Autodesk Inventor part; units mm, degrees
ref_plane "Work Plane1" through (1.525, 0, 0) normal (0, 0, 1) x (1, 0, 0)
ref_plane "YZ Plane" through (0, 0, 0) normal (1, 0, 0) x (0, 1, 0)
ref_plane "XZ Plane" through (0, 0, 0) normal (0, 1, 0) x (-1, 0, 0)
sketch "Sketch1" plane through (0, 0, 0) normal (0, 0, 1) x (1, 0, 0)
  line L0 (0, 10) -> (80, 10)
  line L1 (80, 10) -> (80, 0)
  line L2 (80, 0) -> (0, 0)
  line L3 (-16, 0) -> (96, 0)
  line L4 (0, -2) -> (0, 12)
  line L5 (0, 10) -> (0, 0)
  dimension "d2" = 20
  dimension "d59" = 80
revolve "Body" add sketch "Sketch1" angle 360 about axis through (80, 0, 0) along (-1, 0, 0)
sketch "Sketch2" plane through (0, 0, 0) normal (-1, 0, 0) x (0, 0, 1)
  line L0 (0, 17.3205) -> (15, 8.6603)
  line L1 (15, 8.6603) -> (15, -8.6603)
  line L2 (15, -8.6603) -> (0, -17.3205)
  line L3 (0, -17.3205) -> (-15, -8.6603)
  line L4 (-15, -8.6603) -> (-15, 8.6603)
  line L5 (-15, 8.6603) -> (0, 17.3205)
  line L6 (-21, 0) -> (21, 0)
  line L7 (0, 24.2487) -> (0, -24.2487)
  point P0 (0, 0)
  point P1 (0, 0)
  dimension "d11" = 30
extrude "Head" add sketch "Sketch2" along normal blind 13.4
sketch "Sketch4" plane through (0, 0, 0) normal (0, 0, 1) x (1, 0, 0)
  line L0 (-11.6679, 18) -> (-13.4, 15)
  line L1 (-1.1, 0) -> (-0.234, 0)
  line L2 (-16.0332, 0) -> (2.3992, 0)
  line L3 (-13.4, 18) -> (-11.6679, 18)
  line L4 (-13.4, 15) -> (-13.4, 18)
  line L5 (0, 21.6) -> (0, -3.6)
  dimension "d65" = 30
  dimension "d67" = 30
  dimension "d68" = 36
  dimension "d69" = 13.4
revolve "Chamfer1" cut sketch "Sketch4" angle 360 about axis through (-1.1, 0, 0) along (1, 0, 0)
thread "Thread"
chamfer "Chamfer2" distance 1.5336 distance2 1.5337 1 edges at (80, -10, 0) measured on face at (80, -2.8768, 3.7595)
fillet "Fillet" radius 0.8 1 edges at (0, -10, 0)
ref_plane "Work Plane1" through (1.525, 0, 0) normal (0, 0, 1) x (1, 0, 0)
equation "\"d2\" = GD"
equation "\"d59\" = NLG"
equation "\"d11\" = SW"
equation "\"d3\" = KOH"
equation "\"d15\" = GEL"
equation "\"d6\" = -0.5 * SPD + 0.5 * GD"
equation "\"d71\" = RR1"
equation "\"d65\" = SW"
equation "\"d67\" = ANG1"
equation "\"d68\" = 1.2 * SW"
equation "\"d69\" = KOH"
equation "\"NLG\" = 80"
equation "\"GD\" = NND"
equation "\"KOH\" = 13.4"
equation "\"GEL\" = 46"
equation "\"SW\" = 30"
equation "\"SPD\" = NND - 1.2269 * PTC"
equation "\"SD\" = 0"
equation "\"ANG1\" = 30deg"
equation "\"GAL\" = 0.61345 * PTC"
equation "\"GUL\" = 0.61345 * PTC"
equation "\"RR\" = 0.1"
equation "\"RR1\" = 0.8"
equation "\"GD1\" = THREADDIA - 1.2269 * PTC"
equation "\"TOA\" = 30deg"
equation "\"PTC\" = 2.5"
equation "\"KOH1\" = 8.8"
equation "\"E0\" = 1.155 * SW"
properties part number "ANSI B18.2.3.5M - M20 x 2,5 x 80" material "Steel, Mild"
For this review, take the finished solid that the model builds, in its own axes (mm). A direction names the side the tool comes from. Round coordinates to 2 decimals unless told otherwise and drop trailing zeros. Loops run counter-clockwise (first coordinate to the right, second up) from the corner with the lowest first, then second, coordinate; pieces in that order, holes last. Notation, with made-up numbers: (49.5, -23.5) - (95.5, -23.5) arc R32 cw to (95.5, 6.5) - close; hole circle Ø6 at (46, 21). An arc over 180 degrees is marked (long way). One line per question, with ' | ' between items.
Q1. Tool access review of faces 1 (the flat face through (-6.606, -13.051, -7.395)), 2 (the cylindrical face through (40.18, -2.17, -9.76)): name each direction out of +Z, -Z, +X, -X, +Y, -Y from which nothing blocks a thin tool from reaching the whole face with its end or side.
Taken from the geometry:
face 1: -Z, +X, -X, -Y | face 2: +X
Q2. For pin 1 (4 mm diameter, centred on x = 15.5, z = 2, fed in from +Y); pin 2 (4 mm diameter, centred on x = 47, z = 10, fed in from +Y); pin 3 (1.5 mm diameter, centred on x = 57, z = 4.5, fed in from -Y), all flat-tipped, find the tip position at first contact; note any pin that passes through.
Taken from the geometry:
pin 1: stops at y = 10 | pin 2: stops at y = 6 | pin 3: stops at y = -9.27
Q3. Take a section at A-A (x = 47). Give the boundary of the cut face in (y, z), and give its area (3 significant figures).
Taken from the geometry:
outline: circle Ø20 at (0, 0) | area: 314 mm²
Q4. For line 1 along Y through (x, z) = (63, -0.5); line 2 along X through (y, z) = (-9.5, 6.5); line 3 along Z through (x, y) = (69.5, -5), list the stretches that pass through material, from the lowest coordinate up. Write a range as [from, to].
Taken from the geometry:
line 1: y = [-9.99, 9.99] | line 2: x = [-13.4, 0] | line 3: z = [-8.66, 8.66]
